from build123d import *

# Parameters (mm, degrees)
SALIENTE_EXTRUIR1_DEPTH = 10
CROQUIS2_R              = 1.75
CORTAR_EXTRUIR1_DEPTH   = 92.569427212
CROQUIS3_W              = 3
CROQUIS3_H              = 13.6
SALIENTE_EXTRUIR2_DEPTH = 15
CHAFL_N1_SIZE           = 10
CHAFL_N1_SIZE2          = 2.679491924
REDONDEO1_R             = 3
CROQUIS4_W              = 166.722641079
CROQUIS4_H              = 47.037936504
CORTAR_EXTRUIR2_DEPTH   = 93.22299515


with BuildPart() as part:
    # Croquis1 → Saliente-Extruir1 (new body)
    with BuildSketch(Plane.XY):
        Polygon((-90, -6.8), (-90, -1.8), (-65, -1.8), (-65, 1.8), (-90, 1.8), (-90, 6.8), (90, 6.8), (90, 1.8), (65, 1.8), (65, -1.8), (90, -1.8), (90, -6.8), align=None)
    extrude(amount=SALIENTE_EXTRUIR1_DEPTH)

    # Croquis2 → Cortar-Extruir1 (cut, through all)
    with BuildSketch(Plane(origin=(0, 6.8, 0), x_dir=(1, 0, 0), z_dir=(0, 1, 0))):
        with BuildLine():
            ThreePointArc((-86.15, -10), (-89.972889442, -5), (-86.15, 0))
            Line((-86.15, 0), (-90, 0))
            Line((-90, 0), (-90, -10))
            Line((-90, -10), (-86.15, -10))
        make_face()
        with BuildLine():
            Line((86.15, -10), (90, -10))
            Line((90, -10), (90, 0))
            Line((90, 0), (86.15, 0))
            ThreePointArc((86.15, 0), (89.972889442, -5), (86.15, -10))
        make_face()
        with BuildLine():
            Line((71.15, -5), (-71.15, -5))
            ThreePointArc((-71.15, -5), (-72.786720767, -8.363279233), (-76.15, -10))
            Line((-76.15, -10), (76.15, -10))
            ThreePointArc((76.15, -10), (72.786720767, -8.363279233), (71.15, -5))
        make_face()
        with Locations(Location((81.15, -5, 0), (0, 0, 270))):
            Circle(CROQUIS2_R)
    extrude(amount=-CORTAR_EXTRUIR1_DEPTH, mode=Mode.SUBTRACT)

    # Croquis3 → Saliente-Extruir2 (add)
    with BuildSketch(Plane(origin=(0, 0, 0), x_dir=(-1, 0, 0), z_dir=(0, 0, -1))):
        with Locations((-61.5, 0)):
            Rectangle(CROQUIS3_W, CROQUIS3_H)
        with Locations((61.5, 0)):
            Rectangle(CROQUIS3_W, CROQUIS3_H)
    extrude(amount=SALIENTE_EXTRUIR2_DEPTH)

    # Chaflán1
    chafl_n1_edges = [part.edges().sort_by_distance(p)[0] for p in [
        (0, -6.8, 0),
    ]]
    chafl_n1_side = [part.faces().sort_by_distance(p)[0] for p in [
        (0, 0, 0),
    ]]
    chamfer(chafl_n1_edges, length=CHAFL_N1_SIZE, length2=CHAFL_N1_SIZE2, reference=chafl_n1_side[0])

    # Redondeo1
    redondeo1_edges = [part.edges().sort_by_distance(p)[0] for p in [
        (61.5, 6.8, -15),
        (61.5, -6.8, -15),
        (-61.5, 6.8, -15),
        (-61.5, -6.8, -15),
    ]]
    fillet(redondeo1_edges, radius=REDONDEO1_R)

    # Croquis4 → Cortar-Extruir2 (cut, through all)
    with BuildSketch(Plane(origin=(0, -6.8, 0), x_dir=(-1, 0, 0), z_dir=(0, -1, 0))):
        with Locations((23.36132054, -0.816815002)):
            Rectangle(CROQUIS4_W, CROQUIS4_H)
    extrude(amount=-CORTAR_EXTRUIR2_DEPTH, mode=Mode.SUBTRACT)


solid = part.part
Check sheet for the modelled part. Datum: model origin and axes. Units: mm. A direction names the side the tool comes from. Give positions to 0.01 mm unless a question says otherwise; leave off trailing zeros. Loops run counter-clockwise (first coordinate to the right, second up) from the corner with the lowest first, then second, coordinate; pieces in that order, holes last. Notation, with made-up numbers: M -39,-26.5 L -11,-26.5 A20 ccw -11,1.5 Z; hole C -24.75,-6.75 d3. An arc over 180 degrees is marked long. Use a Markdown table: item, result. Add a question column.
Q1. Scan lines: line 1 along Z through (x, y) = (81.15, 4.25); line 2 along Y through (x, z) = (70, 4.25); line 3 along Z through (x, y) = (63.5, 1.5). Record each from-to range of solid material in increasing order. Write a range as [from, to].
Q2. Sectioned sample at C-C, the plane z = 6. Record the cut outline in (x, y), then the cut area to 3 significant figures.
Q3. Mould release check, pull along Y, two halves, no side actions. Record for faces 5 (the flat face through (78, 1.8, 5)), 6 (the flat face through (75, 6.8, 4)), 7 (the flat face through (65, 0, 2)), 8 (the flat face through (60, 0, -5)): pulls with the +Y half, pulls with the -Y half, needs draft (parallel to the pull), parting line crosses it, or undercut.
Q4. Go/stop test with flat-tipped pins: pin 1 (8 mm diameter, centred on x = 72, y = 1, fed in from +Z); pin 2 (4 mm diameter, centred on y = 2.5, z = -7, fed in from +X); pin 3 (3.5 mm diameter, centred on x = 63.5, y = 0.5, fed in from +Z). Record where each tip stops, or that it passes through.
Q5. Sectioned sample at A-A, the plane x = 69.5. Record the cut outline in (y, z).
Q6. Sectioned sample at D-D, the plane y = 4.25. Record the cut outline in (x, z), then the cut area to 3 significant figures.
Q7. Tool access check on faces 1 (the flat face through (64, 0, 5)), 2 (the flat face through (77, -1.8, 5)), 3 (the flat face through (75, 3, 0)), 4 (the cylindrical face through (61.48, -5.94, -14.1)). Record the directions out of +Z, -Z, +X, -X, +Y, -Y that give a thin tool (end or side, any length) a straight path to the whole face; none if there is none.
Q8. Sectioned sample at B-B, the plane x = 81.15. Record the cut outline in (y, z), then the cut area to 3 significant figures.
Verdict:
| question | item | result |
|---|---|---|
| 1 | line 1 | [0, 3.25], [6.75, 10] |
| 1 | line 2 | [-6.8, -1.8], [1.8, 6.8] |
| 1 | line 3 | [0, 5] |
| 2 | outline | M 71.36,-6.8 L 79.71,-6.8 L 79.71,-1.8 L 71.36,-1.8 Z; M 71.36,1.8 L 79.71,1.8 L 79.71,6.8 L 71.36,6.8 Z; M 82.59,-6.8 L 89.88,-6.8 L 89.88,-1.8 L 82.59,-1.8 Z; M 82.59,1.8 L 89.88,1.8 L 89.88,6.8 L 82.59,6.8 Z |
| 2 | area | 156 mm^2 |
| 3 | face 5 | undercut |
| 3 | face 6 | pulls with the +Y half |
| 3 | face 7 | undercut |
| 3 | face 8 | needs draft |
| 4 | pin 1 | z = 9.97 |
| 4 | pin 2 | x = 63 |
| 4 | pin 3 | z = 5 |
| 5 | outline | M -6.8,0 L -1.8,0 L -1.8,5 L -6.8,5 Z; M 1.8,0 L 6.8,0 L 6.8,5 L 1.8,5 Z |
| 6 | outline | M 60,-14.97 L 63,-14.97 L 63,0 L 86.15,0 A5.18 ccw 86.15,10 L 76.15,10 A5.73 ccw 71.15,5 L 60,5 Z; hole C 81.15,5 d3.5 |
| 6 | area | 263 mm^2 |
| 7 | face 1 | +Z, -X, +Y, -Y |
| 7 | face 2 | +Z, -Z, +X |
| 7 | face 3 | -Z, +X, +Y, -Y |
| 7 | face 4 | -Z, +X, -X, -Y |
| 8 | outline | M -6.8,0 L -1.8,0 L -1.8,3.25 L -6.8,3.25 Z; M -6.8,6.75 L -1.8,6.75 L -1.8,10 L -6.8,10 Z; M 1.8,0 L 6.8,0 L 6.8,3.25 L 1.8,3.25 Z; M 1.8,6.75 L 6.8,6.75 L 6.8,10 L 1.8,10 Z |
| 8 | area | 65.0 mm^2 |
